Part print with two shaded views. Sizes in mm from the minimum x, y, z corner. A direction names the side the tool comes from. Coordinates: 2 decimals unless noted, no trailing zeros. Order: outer loops, then holes, each group sorted by start corner. A loop starts at its lowest first (then second) coordinate and runs counter-clockwise, first axis right, second up. Notation, with made-up numbers: (57, 51.5) - (115, 51.5) arc R27 cw to (115, 88.5) - close; hole circle Ø9 at (-19.5, -9.75). An arc over 180 degrees is marked (long way). Write each question's results on one line, items separated by ' | '. Start each with the question number.
Q1. Pin check, flat tips, straight feed: P1, Ø4, axis at x = 35, y = 12.5, coming from the +Z side; P2, Ø3, axis at y = 20.5, z = 10, coming from the +X side; P3, Ø2, axis at x = 18, z = 16.5, coming from the +Y side. Stop position of each tip, or through.
Q2. Band-saw the part on C-C, the plane x = 5. Write the cut outline in (y, z).
Q3. Which spindle directions (+Z, -Z, +X, -X, +Y, -Y) get a long thin tool onto all of the face, cutting with end or side? Do the marked faces 1 and 2. Say none if no direction does.
Q4. Wall check: probe 1 along Y at (x, z) = (35, 1.25); probe 2 along Z at (x, y) = (2.5, 10.5); probe 3 along Y at (x, z) = (25, 5.5). Give the ranges that are in metal, low to high.
Q5. Band-saw the part on A-A, the plane y = 12.5. Write the cut outline in (x, z), then the cut area to 3 significant figures.
Q6. Band-saw the part on B-B, the plane x = 20. Write the cut outline in (y, z).
Q7. Band-saw the part on D-D, the plane z = 13.75. Write the cut outline in (x, y), then the cut area to 3 significant figures.
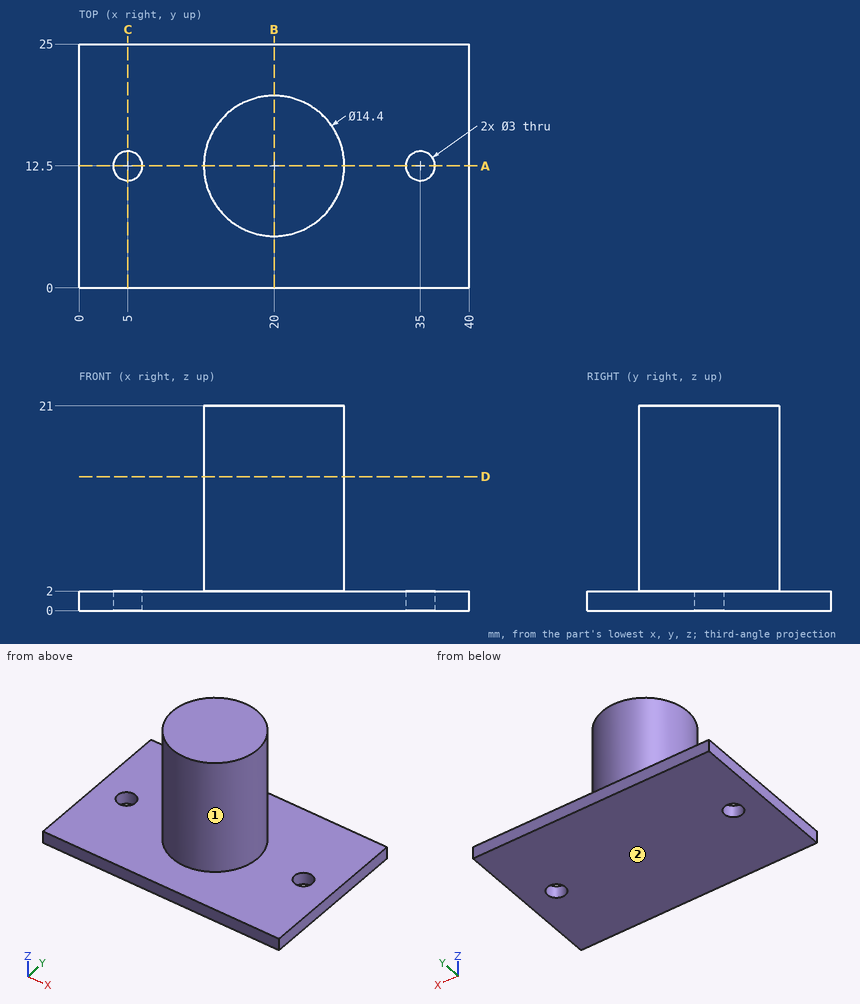
Results below:
1) P1: stops at z = 2 | P2: stops at x = 23.1 | P3: stops at y = 19.63
2) outline: (0, 0) - (11, 0) - (11, 2) - (0, 2) - close; (14, 0) - (25, 0) - (25, 2) - (14, 2) - close
3) face 1: +Z | face 2: -Z, +X, -X, +Y, -Y
4) probe 1: y = 0 to 11, 14 to 25 | probe 2: z = 0 to 2 | probe 3: y = 7.32 to 17.68
5) outline: (0, 0) - (3.5, 0) - (3.5, 2) - (0, 2) - close; (6.5, 0) - (33.5, 0) - (33.5, 2) - (27.2, 2) - (27.2, 21) - (12.8, 21) - (12.8, 2) - (6.5, 2) - close; (36.5, 0) - (40, 0) - (40, 2) - (36.5, 2) - close | area: 342 mm²
6) outline: (0, 0) - (25, 0) - (25, 2) - (19.7, 2) - (19.7, 21) - (5.3, 21) - (5.3, 2) - (0, 2) - close
7) outline: circle Ø14.4 at (20, 12.5) | area: 163 mm²
